Could you check a few things on this model? Use its own coordinates, in mm. Face numbers are marked on the shaded views. A direction names the side the tool comes from. Round coordinates to 2 decimals unless told otherwise and drop trailing zeros. Write each loop counter-clockwise with the first axis right and the second up, starting at its lowest first coordinate (ties: lowest second). Pieces come first, ordered by that corner, then holes. Notation, with made-up numbers: M -19,-18 L -6,-18 A14 cw -6,-1 Z; hole C -10.5,79.25 d3. An arc over 180 degrees is marked long. One line per item, written item: value. Start each with the question number.
(1) If I drill on L1, parallel to Y at x = -64, z = 44; L2, parallel to Y at x = 26.5, z = 13; L3, parallel to Z at x = 6, y = -12, over which ranges is the centre line in solid material (lowest first)?
(2) I want a section at B-B on y = 34.5. Please give me the cut outline in (x, z).
(3) I'm going to push flat-ended pins straight in: pin 1 Ø5 at (y, z) = (-9.5, 6) entering from +X; pin 2 Ø12.5 at (y, z) = (-43, 34.5) entering from +X; pin 3 Ø4 at (y, z) = (-2.5, 33) entering from +X; pin 4 Ø9.5 at (y, z) = (30.31, 12.6) entering from +X. Where does each tip first touch, or does it pass through?
(4) Thinking about a two-plate mould opening in Y: for the marked faces 1, 2 and 3, which applies, released by +Y, released by -Y, zero draft, split by the parting line, or undercut?
(5) Which directions (+Z, -Z, +X, -X, +Y, -Y) give clear straight access to the entire face, cutting with the end or side of a thin tool? Please do the marked faces 4 and 5.
(6) I want a section at C-C on x = -59.5. Please give me the cut outline in (y, z).
(7) I want a section at D-D on y = -31. Please give me the cut outline in (x, z).
(8) I want a section at A-A on z = 16.5. Please give me the cut outline in (x, y).
```python
from build123d import *

# Parameters (mm, degrees)
F0_W     = 172.6877242327
F0_H     = 103.2821238041
F1_DEPTH = 61.722
F2_R     = 7.7359676361
F2_R_2   = 7.3409655567
F2_R_3   = 7.5923806125
F2_R_4   = 7.7547702854
F3_DEPTH = 324.104
F5_DEPTH = 152.4
F6_W     = 64.3570628017
F6_H     = 25.3581311554
F7_DEPTH = 75.438
F8_W     = 16.7872086167
F8_H     = 7.7908643157
F9_DEPTH = 109.728


with BuildPart() as f1:
    # F0 (on Top) → F1 (new body)
    with BuildSketch(Plane.XY):
        Rectangle(F0_W, F0_H)
    extrude(amount=F1_DEPTH)

    # F2 (on face) → F3 (cut)
    with BuildSketch(Plane.YZ.offset(86.3438621163)):
        with Locations((30.3141865879, 44.6238219738)):
            Circle(F2_R)
        with Locations((-9.4450721517, 44.6238219738)):
            Circle(F2_R_2)
        with Locations((-9.4450721517, 12.600524351)):
            Circle(F2_R_3)
        with Locations((30.3141865879, 12.600524351)):
            Circle(F2_R_4)
    extrude(amount=-F3_DEPTH, mode=Mode.SUBTRACT)

    # F4 (on face) → F5 (cut)
    with BuildSketch(Plane.XZ.offset(51.641061902)):
        Polygon((86.3438621163, 61.722), (0, 61.722), (86.3438621163, 0), align=None)
    extrude(amount=-F5_DEPTH, mode=Mode.SUBTRACT)

    # F6 (on face) → F7 (cut)
    with BuildSketch(Plane(origin=(0, 0, 0), x_dir=(1, 0, 0), z_dir=(0, 0, -1))):
        with Locations((54.1653307155, 38.9619963244)):
            Rectangle(F6_W, F6_H)
    extrude(amount=-F7_DEPTH, mode=Mode.SUBTRACT)

    # F8 (on face) → F9 (cut)
    with BuildSketch(Plane(origin=(-86.3438621163, 0, 0), x_dir=(0, -1, 0), z_dir=(-1, 0, 0))):
        with Locations((0, 57.8265678421)):
            Rectangle(F8_W, F8_H)
    extrude(amount=-F9_DEPTH, mode=Mode.SUBTRACT)


solid = f1.part
```
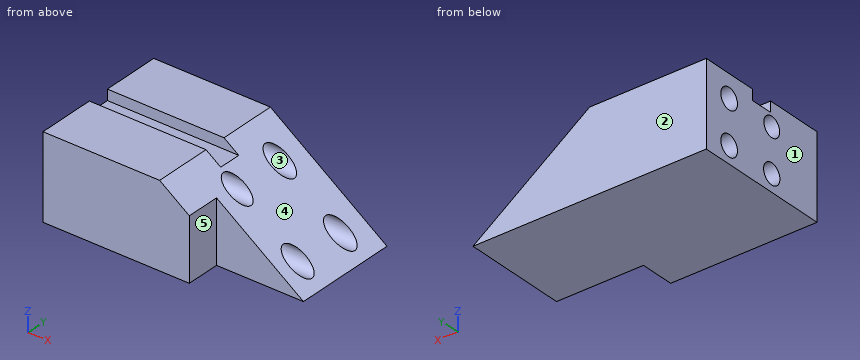
Found:
1. L1: y = -51.64 to -16.76, -2.13 to 22.6, 38.02 to 51.64
1. L2: y = -26.28 to -17.03, -1.86 to 22.57, 38.06 to 51.64
1. L3: z = 0 to 5.45, 19.75 to 37.74, 51.51 to 57.43
2. outline: M -86.34,0 L 86.34,0 L 77.85,6.07 L -86.34,6.07 Z; M -86.34,19.13 L 59.58,19.13 L 33.02,38.12 L -86.34,38.12 Z; M -86.34,51.13 L 14.82,51.13 L 0,61.72 L -86.34,61.72 Z
3. pin 1: stops at x = 81.45
3. pin 2: stops at x = 21.99
3. pin 3: stops at x = 42.98
3. pin 4: passes through
4. face 1: zero draft
4. face 2: released by +Y
4. face 3: undercut
5. face 4: +Z, +X, +Y, -Y
5. face 5: +Z, -Z, +X, -Y
6. outline: M -51.64,0 L 51.64,0 L 51.64,61.72 L 8.39,61.72 L 8.39,53.93 L -8.39,53.93 L -8.39,61.72 L -51.64,61.72 Z; hole C -9.45,12.6 d15.18; hole C -9.45,44.62 d14.68; hole C 30.31,12.6 d15.51; hole C 30.31,44.62 d15.47
7. outline: M -86.34,0 L 21.99,0 L 21.99,46 L 0,61.72 L -86.34,61.72 Z
8. outline: M -86.34,-51.64 L 21.99,-51.64 L 21.99,-26.28 L 63.26,-26.28 L 63.26,-15.96 L -86.34,-15.96 Z; M -86.34,-2.93 L 63.26,-2.93 L 63.26,23.61 L -86.34,23.61 Z; M -86.34,37.02 L 63.26,37.02 L 63.26,51.64 L -86.34,51.64 Z
